Autodesk Inventor part; units mm, degrees
ref_plane "YZ Plane" through (0, 0, 0) normal (1, 0, 0) x (0, 1, 0)
ref_plane "XZ Plane" through (0, 0, 0) normal (0, 1, 0) x (-1, 0, 0)
ref_plane "XY Plane" through (0, 0, 0) normal (0, 0, 1) x (1, 0, 0)
sketch "Boceto1" plane through (0, 0, 0) normal (0, 1, 0) x (-1, 0, 0)
  line L0 (6.2354, 0) -> (3.1177, -5.4)
  line L1 (3.1177, -5.4) -> (-3.1177, -5.4)
  line L2 (-3.1177, -5.4) -> (-6.2354, 0)
  line L3 (-6.2354, 0) -> (-3.1177, 5.4)
  line L4 (-3.1177, 5.4) -> (3.1177, 5.4)
  line L5 (3.1177, 5.4) -> (6.2354, 0)
  circle A0 centre (0, 0) radius 5.4
  line L6 (4.3879, 0) -> (2.1939, -3.8)
  line L7 (2.1939, -3.8) -> (-2.1939, -3.8)
  line L8 (-2.1939, -3.8) -> (-4.3879, 0)
  line L9 (-4.3879, 0) -> (-2.1939, 3.8)
  line L10 (-2.1939, 3.8) -> (2.1939, 3.8)
  line L11 (2.1939, 3.8) -> (4.3879, 0)
  dimension "d0" = 10.8
  dimension "d4" = 1.6
extrude "Extrusión1" add sketch "Boceto1" along normal blind 3
sketch "Boceto2" plane through (0, 3, 0) normal (0, 1, 0) x (1, 0, 0)
  line L0 (8.9124, 8.7156) -> (4, 8.7156)
  line L1 (4, 8.7156) -> (4, -10.3861)
  line L2 (4, -10.3861) -> (8.9124, -10.3861)
  line L3 (8.9124, -10.3861) -> (8.9124, 8.7156)
  point P0 (0, 0)
  dimension "d22" = 4
extrude "Extrusión2" cut sketch "Boceto2" against normal through all
fillet "Empalme1" radius 1 4 edges at (3.1177, 1.5, -5.4) (3.1177, 1.5, 5.4) (-3.1177, 1.5, 5.4) (-3.1177, 1.5, -5.4)
fillet "Empalme2" radius 0.7 2 edges at (4, 1.5, -0.6718) (4, 1.5, 0.6718)
sketch "Boceto3" plane through (0, 3, 0) normal (0, 1, 0) x (1, 0, 0)
  line L0 (-23.3379, 5.4) -> (-4.3879, 5.4)
  line L1 (-4.3879, 5.4) -> (-4.3879, -5.4)
  line L2 (-4.3879, -5.4) -> (-23.3379, -5.4)
  line L3 (-23.3379, -5.4) -> (-23.3379, 5.4)
  line L4 (-23.3379, 5.4) -> (-4.3879, -5.4) construction
  line L5 (-4.3879, 5.4) -> (-23.3379, -5.4) construction
  line L6 (2.6938, -2.9342) -> (2.1939, -3.8)
  line L7 (2.1939, -3.8) -> (-2.1939, -3.8)
  line L8 (-2.1939, -3.8) -> (-4.3879, 0)
  line L9 (-4.3879, 0) -> (-2.1939, 3.8)
  line L10 (-2.1939, 3.8) -> (2.1939, 3.8)
  line L11 (2.1939, 3.8) -> (2.6938, 2.9342)
  arc A0 (3.4064, 4.9) -> (2.5403, 5.4) centre (2.5403, 4.4) ccw
  line L12 (2.5403, 5.4) -> (-2.5403, 5.4)
  arc A1 (-2.5403, 5.4) -> (-3.4064, 4.9) centre (-2.5403, 4.4) ccw
  line L13 (-3.4064, 4.9) -> (-6.2354, 0)
  line L14 (-6.2354, 0) -> (-3.4064, -4.9)
  arc A2 (-3.4064, -4.9) -> (-2.5403, -5.4) centre (-2.5403, -4.4) ccw
  line L15 (-2.5403, -5.4) -> (2.5403, -5.4)
  arc A3 (2.5403, -5.4) -> (3.4064, -4.9) centre (2.5403, -4.4) ccw
  line L16 (-4.3879, 5.4) -> (-0.8083, 5.4)
  line L17 (-0.8083, 5.4) -> (-0.8083, -5.4)
  line L18 (-0.8083, -5.4) -> (-4.3879, -5.4)
  line L19 (-4.3879, -5.4) -> (-4.3879, 5.4)
  circle A4 centre (-25, 0) radius 3.6
  circle A5 centre (-25, 0) radius 5.65
  line L20 (3.4064, -4.9) -> (4, -3.8718)
  line L21 (4, 3.8718) -> (3.4064, 4.9)
  line L22 (4, -3.8718) -> (4, -3.2842)
  line L23 (4, 3.2842) -> (4, 3.8718)
  arc A6 (4, -3.2842) -> (2.6938, -2.9342) centre (3.3, -3.2842) ccw
  arc A7 (2.6938, 2.9342) -> (4, 3.2842) centre (3.3, 3.2842) ccw
  point P0 (0, 0)
  point P1 (-13.8629, 0)
  point P2 (-13.8629, 0)
  point P3 (-13.8629, 0)
  point P4 (-2.5403, -5.4)
  point P5 (-2.5403, 5.4)
  point P6 (-23.3379, 5.4)
  point P7 (-2.8868, 4)
  point P8 (-4.3879, 3.2)
  point P9 (-4.3879, -3.2)
  point P10 (-23.3379, 5.4)
  point P11 (-0.8083, -3.8)
  point P12 (-0.8083, 3.8)
  point P13 (-0.8083, 5.4)
  dimension "d12" = 11.3
  dimension "d10" = 25
  dimension "d11" = 7.2
extrude "Extrusión3" add sketch "Boceto3" against normal up to surface (3 mm away) contours A5 L3 A4 | L0 L1 L13 L14 L2 A5 | L3 A4 A5 | L16 A1 L13 L1 | L1 L14 A2 L18
sketch "Boceto4" plane through (0, 3, 0) normal (0, 1, 0) x (1, 0, 0)
  arc A0 (-23.3379, 5.4) -> (-4, 5.4) centre (-13.669, 33.7991) ccw
  line L0 (-23.3379, -5.4) -> (2.5403, -5.4)
  arc A1 (-4, -5.4) -> (-23.3379, -5.4) centre (-13.669, -33.7991) ccw
  circle A2 centre (-25, 0) radius 3.6
  line L1 (2.6938, -2.9342) -> (2.1939, -3.8)
  line L2 (2.1939, -3.8) -> (-2.1939, -3.8)
  line L3 (-2.1939, -3.8) -> (-4.3879, 0)
  line L4 (-4.3879, 0) -> (-2.1939, 3.8)
  line L5 (-2.1939, 3.8) -> (2.1939, 3.8)
  line L6 (2.1939, 3.8) -> (2.6938, 2.9342)
  arc A3 (3.4064, 4.9) -> (2.5403, 5.4) centre (2.5403, 4.4) ccw
  line L7 (2.5403, 5.4) -> (-23.3379, 5.4)
  arc A4 (-23.3379, 5.4) -> (-23.3379, -5.4) centre (-25, 0) ccw
  line L8 (-23.3379, -5.4) -> (2.5403, -5.4)
  arc A5 (2.5403, -5.4) -> (3.4064, -4.9) centre (2.5403, -4.4) ccw
  line L9 (3.4064, -4.9) -> (4, -3.8718)
  line L10 (4, 3.8718) -> (3.4064, 4.9)
  line L11 (4, 3.2842) -> (4, 3.8718)
  line L12 (4, -3.8718) -> (4, -3.2842)
  arc A6 (4, -3.2842) -> (2.6938, -2.9342) centre (3.3, -3.2842) ccw
  arc A7 (2.6938, 2.9342) -> (4, 3.2842) centre (3.3, 3.2842) ccw
  line L13 (2.5403, 5.4) -> (-23.3379, 5.4)
  point P0 (0, 0)
  point P1 (-4, 5.4)
  dimension "d16" = 4
  dimension "d18" = 30
extrude "Extrusión4" cut sketch "Boceto4" against normal through all contours L7 A0 | A1 L0
fillet "Empalme4" radius 3 2 edges at (-23.3379, 1.5, -5.4) (-23.3379, 1.5, 5.4)
properties part number "ShortLink"
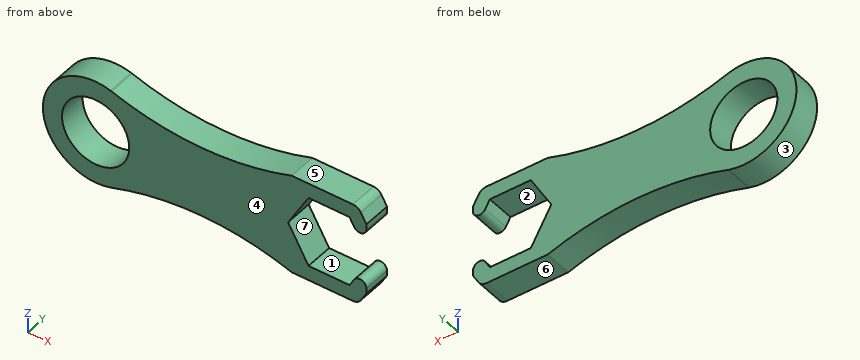
Design review of the part built by this model. Coordinates are the model's own, in mm. Face numbers are marked on the shaded views. A direction names the side the tool comes from. Give positions to 0.01 mm unless a question says otherwise; leave off trailing zeros. Write each loop counter-clockwise with the first axis right and the second up, starting at its lowest first coordinate (ties: lowest second). Pieces come first, ordered by that corner, then holes. Notation, with made-up numbers: M -36,65.5 L 23,65.5 A22 cw 23,104.5 Z; hole C 18,19.25 d1. An arc over 180 degrees is marked long. Answer as a JSON object with one key per item and string values. Group by question number.
1) Tool access review of the marked faces 5, 6 and 7: name each direction out of +Z, -Z, +X, -X, +Y, -Y from which nothing blocks a thin tool from reaching the whole face with its end or side.
2) We need section D-D (x = -6.5). Give the boundary of the cut face in (y, z), and give its area (3 significant figures).
3) We need section C-C (z = -2). Give the boundary of the cut face in (x, y), and give its area (3 significant figures).
4) Mouldability with a two-part tool opening along X and no side actions: class the marked faces 1, 2, 3 and 4 as released by +X, released by -X, zero draft, split by the parting line, or undercut.
5) For line 1 along Z through (x, y) = (-1.5, 1.2); line 2 along Z through (x, y) = (-25, 1.7); line 3 along X through (y, z) = (1.1, 1.5), list the stretches that pass through material, from the lowest coordinate up.
6) We need section B-B (x = -25). Give the boundary of the cut face in (y, z).
7) Clearance check with flat-ended pins moving along their axes: pin 1 Ø1.5 at (x, y) = (-2.5, 1) entering from -Z; pin 2 Ø1.5 at (x, z) = (-24.5, -1.5) entering from -Y. State where each tip first meets the part, or that it passes through.
8) We need section A-A (y = 0.65). Give the boundary of the cut face in (x, z).
Answer key:
{
 "1": {"face 5": "+Z, +X, +Y, -Y", "face 6": "-Z, +X, +Y, -Y", "face 7": "+Y, -Y"},
 "2": {"outline": "M 0,-4.67 L 3,-4.67 L 3,4.67 L 0,4.67 Z", "area": "28.0 mm²"},
 "3": {"outline": "M -30.28,0 L -27.99,0 L -27.99,3 L -30.28,3 Z; M -22.01,0 L -3.23,0 L -3.23,3 L -22.01,3 Z", "area": "63.2 mm²"},
 "4": {"face 1": "undercut", "face 2": "undercut", "face 3": "split by the parting line", "face 4": "zero draft"},
 "5": {"line 1": "z = -5.4 to -3.8, 3.8 to 5.4", "line 2": "z = -5.65 to -3.6, 3.6 to 5.65", "line 3": "x = -30.45 to -28.27, -21.73 to -3.52"},
 "6": {"outline": "M 0,-5.65 L 3,-5.65 L 3,-3.6 L 0,-3.6 Z; M 0,3.6 L 3,3.6 L 3,5.65 L 0,5.65 Z"},
 "7": {"pin 1": "stops at z = -5.4", "pin 2": "passes through"},
 "8": {"outline": "M -23.41,-5.42 A3 ccw -23.29,-5.38 A30 cw -4,-5.4 L 2.54,-5.4 A1 ccw 3.41,-4.9 L 4,-3.87 L 4,-3.28 A0.7 ccw 2.69,-2.93 L 2.19,-3.8 L -2.19,-3.8 L -4.39,0 L -2.19,3.8 L 2.19,3.8 L 2.69,2.93 A0.7 ccw 4,3.28 L 4,3.87 L 3.41,4.9 A1 ccw 2.54,5.4 L -4,5.4 A30 cw -23.29,5.38 A3 ccw -23.41,5.42 A5.65 ccw long Z; hole C -25,0 d7.2"}
}
